Can you work these out from the model? Positions are in its coordinate system, mm. Face numbers are marked on the shaded views. A direction names the side the tool comes from. Coordinates: 2 decimals unless noted, no trailing zeros. Order: outer loops, then holes, each group sorted by start corner. A loop starts at its lowest first (then second) coordinate and runs counter-clockwise, first axis right, second up. Notation, with made-up numbers: (-12, -39) - (34, -39) arc R23 ccw to (34, -30) - close; hole circle Ø11 at (8.25, 17). An arc over 180 degrees is marked (long way). Return JSON: item names as keys, results as strings. Group by question number.
1) For pin 1 Ø5 at (y, z) = (9.5, 7.5) entering from -X; pin 2 Ø4 at (x, z) = (-7, 7.5) entering from -Y; pin 3 Ø7.5 at (y, z) = (3, 13) entering from +X, each with a flat end and sliding along its axis, tell me the tip position at first contact or that it passes through.
2) Imagine slicing it at A-A (z = 16). Write out the boundary of the cut face in (x, y).
3) Imagine slicing it at C-C (x = -14.5). Write out the boundary of the cut face in (y, z).
4) Which directions (+Z, -Z, +X, -X, +Y, -Y) give clear straight access to the entire face, cutting with the end or side of a thin tool? Please do the marked faces 1, 2, 3 and 4.
5) If I drill on line 1 along Y through (x, z) = (-20.5, 17.25); line 2 along X through (y, z) = (-19, 22); line 3 along Y through (x, z) = (-34, 16.75), over which ranges is the centre line in solid material (lowest first)?
6) Imagine slicing it at B-B (y = 31). Write out the boundary of the cut face in (x, z), and give its area (3 significant figures).
```python
from build123d import *

# Parameters (mm, degrees)
F1_DEPTH = 25.4


# Not quite as in the source:
# - a feature names something its author has since deleted; it is built from what else it names


with BuildPart() as f1:
    # F0 (on Top) → F1 (new body)
    with BuildSketch(Plane.XY):
        Polygon((-32.0039994973, 49.1343741807), (-39.6239994973, 49.1343741807), (-39.6239994973, 41.5143741807), (-39.6239994973, -27.0656258193), (-34.8614994973, -27.0656258193), (-34.8614994973, 44.3718741807), (36.5760005027, 44.3718741807), (36.5760005027, 49.1343741807), align=None)
        with BuildLine():
            Line((-39.6239994973, 41.5143741807), (-39.6239994973, 49.1343741807))
            Line((-39.6239994973, 49.1343741807), (-32.0039994973, 49.1343741807))
            ThreePointArc((-32.0039994973, 49.1343741807), (-42.8727293035, 52.3831039869), (-39.6239994973, 41.5143741807))
        make_face()
    extrude(amount=F1_DEPTH)


solid = f1.part
```
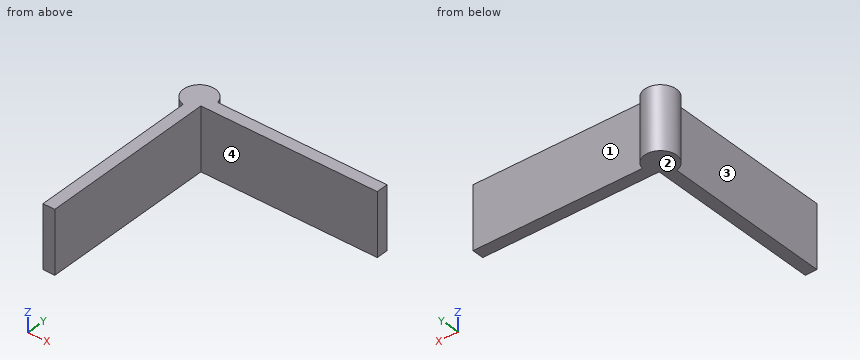
Calculated:
{
 "1": {"pin 1": "x = -39.62", "pin 2": "y = 44.37", "pin 3": "x = -34.86"},
 "2": {"outline": "(-39.62, -27.07) - (-34.86, -27.07) - (-34.86, 44.37) - (36.58, 44.37) - (36.58, 49.13) - (-32, 49.13) arc R6.45 ccw (long way) to (-39.62, 41.51) - close"},
 "3": {"outline": "(44.37, 0) - (49.13, 0) - (49.13, 25.4) - (44.37, 25.4) - close"},
 "4": {"face 1": "+Z, -Z, +X, +Y", "face 2": "-Z, +X, -X, +Y, -Y", "face 3": "+Z, -Z, -X, -Y", "face 4": "+Z, -Z, +X, -Y"},
 "5": {"line 1": "44.37 to 49.13", "line 2": "-39.62 to -34.86", "line 3": "44.37 to 52.61"},
 "6": {"outline": "(-39.62, 0) - (-34.86, 0) - (-34.86, 25.4) - (-39.62, 25.4) - close", "area": "121 mm2"}
}
